Read the model definition and answer for the solid it produces. Units are mm, in the model's axes. A direction names the side the tool comes from. Give positions to 0.01 mm unless a question says otherwise; leave off trailing zeros. Write each loop counter-clockwise with the first axis right and the second up, starting at its lowest first coordinate (ties: lowest second). Pieces come first, ordered by that corner, then holes.
```python
from build123d import *

# Parameters (mm, degrees)
F0_R     = 1.0668
F0_W     = 12.319
F0_H     = 22.5044
F0_R_2   = 1.4732
F1_DEPTH = 3.175


with BuildPart() as f1:
    # F0 (on Top) → F1 (new body)
    with BuildSketch(Plane.XY):
        with BuildLine():
            Line((34.925, 82.804), (34.925, 12.7))
            Line((34.925, 12.7), (-28.575, 12.7))
            Line((-28.575, 12.7), (-28.575, 63.5))
            ThreePointArc((-28.575, 63.5), (-42.045384, 57.920384), (-47.625, 44.45))
            Line((-47.625, 44.45), (-47.625, 12.7))
            ThreePointArc((-47.625, 12.7), (-40.185512, -5.260512), (-22.225, -12.7))
            Line((-22.225, -12.7), (22.225, -12.7))
            ThreePointArc((22.225, -12.7), (40.185512, -5.260512), (47.625, 12.7))
            Line((47.625, 12.7), (47.625, 76.2))
            ThreePointArc((47.625, 76.2), (43.905256, 85.180256), (34.925, 88.9))
            Line((34.925, 88.9), (34.925, 82.804))
        make_face()
        with Locations((-38.1, 4.1656)):
            Circle(F0_R, mode=Mode.SUBTRACT)
        with Locations((-38.1, 18.161)):
            Rectangle(F0_W, F0_H, mode=Mode.SUBTRACT)
        with Locations((-38.1, 32.1564)):
            Circle(F0_R, mode=Mode.SUBTRACT)
        with Locations((-38.1, 50.8)):
            Circle(F0_R_2, mode=Mode.SUBTRACT)
    extrude(amount=F1_DEPTH)


solid = f1.part
```
Item 1: Section B-B (y = 35.5) is taken. Write down the section's boundary in (x, z) (3 decimals), and give its area (3 significant figures).
Result set:
outline: (-47.625, 0) - (-28.575, 0) - (-28.575, 3.175) - (-47.625, 3.175) - close; (34.925, 0) - (47.625, 0) - (47.625, 3.175) - (34.925, 3.175) - close
area: 101 mm2
Item 2: Section A-A (y = 21.5) is taken. Write down the section's boundary in (x, z) (1 decimal).
Result set:
outline: (-47.6, 0) - (-44.3, 0) - (-44.3, 3.2) - (-47.6, 3.2) - close; (-31.9, 0) - (-28.6, 0) - (-28.6, 3.2) - (-31.9, 3.2) - close; (34.9, 0) - (47.6, 0) - (47.6, 3.2) - (34.9, 3.2) - close
Item 3: Find the intervals of material crossed by line 1 along X through (y, z) = (17.5, 2.3) (1 decimal); line 2 along Y through (x, z) = (-38.1, 1.7); line 3 along Y through (x, z) = (-38.5, 0.4), in increasing order.
Result set:
line 1: x = -47.6 to -44.3, -31.9 to -28.6, 34.9 to 47.6
line 2: y = -7.13 to 3.1, 5.23 to 6.91, 29.41 to 31.09, 33.22 to 49.33, 52.27 to 60.95
line 3: y = -6.8 to 3.18, 5.15 to 6.91, 29.41 to 31.17, 33.15 to 49.38, 52.22 to 60.71
Item 4: Section D-D (x = -21) is taken. Write down the section's boundary in (y, z) (3 decimals).
Result set:
outline: (-12.7, 0) - (12.7, 0) - (12.7, 3.175) - (-12.7, 3.175) - close
Item 5: Determine the mould class of faces 1 (the flat face through (0, -12.7, 2)), 2 (the cylindrical face through (-38.29, 52.26, 1.57)), 3 (the flat face through (-44.26, 18, 2)), 4 (the flat face through (47.625, 44, 2)) for opening direction X: pulls with the +X half, pulls with the -X half, needs draft (parallel to the pull), parting line crosses it, or undercut.
Result set:
face 1: needs draft
face 2: undercut
face 3: undercut
face 4: pulls with the +X half
Item 6: Each of these flat-tipped pins is pushed along its axis until it touches: pin 1 Ø3.5 at (x, y) = (-38.1, 50.8) entering from +Z (3 decimals); pin 2 Ø1 at (x, z) = (4.5, 1) entering from +Y; pin 3 Ø1.5 at (x, z) = (33, 2) entering from -Y; pin 4 Ø1 at (y, z) = (53, 1.5) entering from -X. Where does it stop, or does it pass through?
Result set:
pin 1: stops at z = 3.175
pin 2: stops at y = 12.7
pin 3: stops at y = -10.64
pin 4: stops at x = -45.84
Item 7: Section C-C (z = 1.55) is taken. Give the number of separate pieces and of enclosed holes in the cut face, and give its area (3 significant figures).
Result set:
separate pieces: 1
enclosed holes: 4
area: 3,670 mm2
Item 8: Which of the six approach directions +Z, -Z, +X, -X, +Y, -Y give full straight-line access (tool end or side, diameter ignored) to faces 5 (the flat face through (34.925, 51, 2)), 6 (the flat face through (-31.94, 18, 2)), 7 (the cylindrical face through (44.003, 85.081, 1.565))?
Result set:
face 5: +Z, -Z, +Y
face 6: +Z, -Z
face 7: +Z, -Z, +X, +Y
